Verification items for the finished model (mm, model axes). Face numbers are marked on the shaded views. A direction names the side the tool comes from. Round coordinates to 2 decimals unless told otherwise and drop trailing zeros. Write each loop counter-clockwise with the first axis right and the second up, starting at its lowest first coordinate (ties: lowest second). Pieces come first, ordered by that corner, then holes. Notation, with made-up numbers: M 53.5,5 L 87.5,5 A26 ccw 87.5,30 Z; hole C -35,39.5 d1. An arc over 180 degrees is marked long. One line per item, written item: value. Start each with the question number.
Item 1: Draft check along Z on the marked faces 1, 2 and 3. Enter one of: +Z half, -Z half, draft (parallel to the pull), parting line (faces both ways), or undercut.
Item 2: Tool access check on the marked faces 4, 5, 6, 7 and 8. Record the directions out of +Z, -Z, +X, -X, +Y, -Y that give a thin tool (end or side, any length) a straight path to the whole face; none if there is none.
Item 3: Gauge pin test, flat ends, axial feed: pin 1 (8 mm diameter, centred on x = 16, z = -26, fed in from -Y); pin 2 (6 mm diameter, centred on x = 27.5, y = 5, fed in from -Z); pin 3 (3 mm diameter, centred on x = 21, z = -23, fed in from -Y); pin 4 (6 mm diameter, centred on y = 1.5, z = -26, fed in from +X). Record the tip position at first contact, or that the pin passes through.
Item 4: Section check D-D, the plane x = 25. Record the cut outline in (y, z), then the cut area to 3 significant figures.
Item 5: Thickness scan on probe 1 along X at (y, z) = (10.5, -26.75); probe 2 along Z at (x, y) = (26.25, 6.25); probe 3 along X at (y, z) = (13, -14). Record the ranges inside material, lowest first. Write a range as from..to.
Item 6: Section check B-B, the plane z = -27.5. Record the cut outline in (x, y), then the cut area to 3 significant figures.
Item 7: Section check C-C, the plane z = -6.5. Record the cut outline in (x, y), then the cut area to 3 significant figures.
Item 8: Section check A-A, the plane y = 5.25. Record the cut outline in (x, z), then the cut area to 3 significant figures.
from build123d import *

# Parameters (mm, degrees)
BOSS_EXTRUDE1_DEPTH = 30.9
SHELL1_T            = -4
CUT_EXTRUDE1_REACH  = 54.486
SKETCH2_W           = 15
SKETCH2_H           = 22.9
CUT_EXTRUDE2_DEPTH  = 16.9
FILLET1_R           = 5
FILLET2_R           = 1.2
SKETCH4_R           = 5
CUT_EXTRUDE5_DEPTH  = 44.588989435


with BuildPart() as part:
    # Sketch1 → Boss-Extrude1 (new body)
    with BuildSketch(Plane(origin=(0, 0, 0), x_dir=(1, 0, 0), z_dir=(0, 1, 0))):
        Polygon((0, 0), (30, 0), (30, 18.4), (18.4, 18.4), (18.4, 30), (0, 30), align=None)
    extrude(amount=BOSS_EXTRUDE1_DEPTH)

    # Shell1
    shell1_openings = [part.faces().sort_by_distance(p)[0] for p in [
        (9.2, 15.45, -30),
        (30, 15.45, -9.2),
    ]]
    offset(amount=SHELL1_T, openings=shell1_openings, kind=Kind.INTERSECTION)

    # Sketch2 → Cut-Extrude1 (cut, up to next)
    with BuildSketch(Plane.XY, mode=Mode.PRIVATE) as cut_extrude1_sk1:
        with Locations((11.5, 15.45)):
            Rectangle(SKETCH2_W, SKETCH2_H)
    cut_extrude1_tool1 = extrude(cut_extrude1_sk1.sketch, amount=-CUT_EXTRUDE1_REACH, mode=Mode.PRIVATE) & part.part
    add(cut_extrude1_tool1.solids().sort_by_distance((11.5, 15.45, 0))[0], mode=Mode.SUBTRACT)

    # Sketch3 → Cut-Extrude2 (cut)
    with BuildSketch(Plane(origin=(0, 30.9, 0), x_dir=(1, 0, 0), z_dir=(0, 1, 0))):
        Polygon((0, 30), (0, 0), (30, 0), (30, 18.4), (18.4, 18.4), (18.4, 30), align=None)
    extrude(amount=-CUT_EXTRUDE2_DEPTH, mode=Mode.SUBTRACT)

    # Fillet1
    fillet1_edges = [part.edges().sort_by_distance(p)[0] for p in [
        (14.4, 9, -14.4),
        (18.4, 7, -18.4),
    ]]
    fillet(fillet1_edges, radius=FILLET1_R)

    # Fillet2
    fillet2_edges = [part.edges().sort_by_distance(p)[0] for p in [
        (19, 9, -4),
        (19, 9, 0),
        (14.4, 9, -30),
        (30, 9, -14.4),
        (30, 9, -4),
        (4, 9, -30),
        (4, 9, 0),
        (18.4, 7, -30),
        (30, 7, -18.4),
        (30, 7, 0),
        (0, 7, 0),
        (0, 7, -30),
    ]]
    fillet(fillet2_edges, radius=FILLET2_R)

    # Sketch4 → Cut-Extrude5 (cut, through all)
    with BuildSketch(Plane(origin=(0, 4, 0), x_dir=(1, 0, 0), z_dir=(0, 1, 0))):
        with Locations(Location((9.932233047, 9.932233047, 0), (0, 0, 270))):
            Circle(SKETCH4_R)
    extrude(amount=-CUT_EXTRUDE5_DEPTH, mode=Mode.SUBTRACT)


solid = part.part
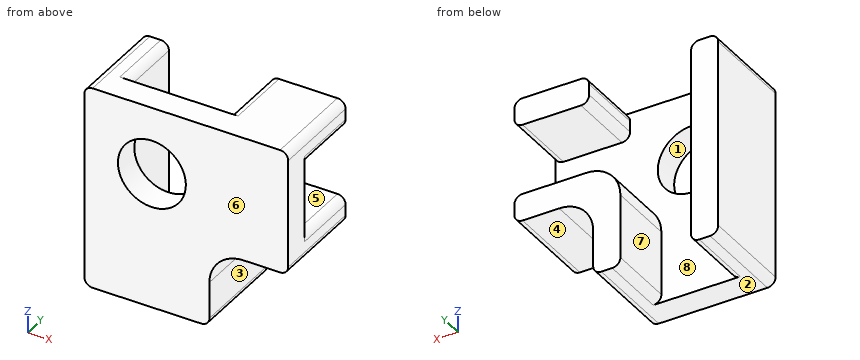
Response values:
1. face 1: undercut
1. face 2: -Z half
1. face 3: draft
2. face 4: -Z, +X, +Y, -Y
2. face 5: +X, +Y
2. face 6: +Z, -Z, +X, -X, -Y
2. face 7: +Z, -Z, +Y
2. face 8: +Y
3. pin 1: stops at y = 0
3. pin 2: stops at z = -18.4
3. pin 3: passes through
3. pin 4: stops at x = 18.42
4. outline: M 0,-18.4 L 14,-18.4 L 14,-14.4 L 4,-14.4 L 4,-4 L 14,-4 L 14,0 L 0,0 Z
4. area: 154 mm2
5. probe 1: x = 0..4, 14.4..18.4
5. probe 2: z = -18.4..-14.4, -4..0
5. probe 3: x = 0..4
6. outline: M 0,0 L 18.4,0 L 18.4,14 L 14.4,14 L 14.4,4 L 4,4 L 4,14 L 0,14 Z
6. area: 154 mm2
7. outline: M 0,0 L 6.3,0 L 6.3,4 L 4,4 L 4,14 L 0,14 Z; M 13.57,0 L 30,0 L 30,4 L 13.57,4 Z
7. area: 131 mm2
8. outline: M 0,-28.8 A1.2 ccw 1.2,-30 L 2.8,-30 A1.2 ccw 4,-28.8 L 4,-1.2 A1.2 ccw 2.8,0 L 1.2,0 A1.2 ccw 0,-1.2 Z; M 14.4,-28.8 A1.2 ccw 15.6,-30 L 17.2,-30 A1.2 ccw 18.4,-28.8 L 18.4,-23.4 A5 cw 23.4,-18.4 L 28.8,-18.4 A1.2 ccw 30,-17.2 L 30,-15.6 A1.2 ccw 28.8,-14.4 L 19.4,-14.4 A5 ccw 14.4,-19.4 Z; M 19,-2.8 A1.2 ccw 20.2,-4 L 28.8,-4 A1.2 ccw 30,-2.8 L 30,-1.2 A1.2 ccw 28.8,0 L 20.2,0 A1.2 ccw 19,-1.2 Z
8. area: 269 mm2
